Here's how the part is built. I have some questions about the finished solid (model axes, mm). Round coordinates to 2 decimals unless told otherwise and drop trailing zeros. Order: outer loops, then holes, each group sorted by start corner. A loop starts at its lowest first (then second) coordinate and runs counter-clockwise, first axis right, second up.
```python
from build123d import *

# Parameters (mm, degrees)
SKETCH_R        = 17.65
SKETCH_R_2      = 15.4
PAD_DEPTH       = 30
CHAMFER_SIZE    = 1.4
CHAMFER001_SIZE = 1.4


with BuildPart() as part:
    # Sketch → Pad (new body)
    with BuildSketch(Plane.XY):
        Circle(SKETCH_R)
        Circle(SKETCH_R_2, mode=Mode.SUBTRACT)
    extrude(amount=PAD_DEPTH)

    # Chamfer
    chamfer_edges = [part.edges().sort_by_distance(p)[0] for p in [
        (-17.65, 0, 30),
    ]]
    chamfer(chamfer_edges, length=CHAMFER_SIZE)

    # Chamfer001
    chamfer001_edges = [part.edges().sort_by_distance(p)[0] for p in [
        (-15.4, 0, 0),
    ]]
    chamfer(chamfer001_edges, length=CHAMFER001_SIZE)


solid = part.part
```
1) I need wall thicknesses on line 1 (Y direction, x = 0, z = 10); line 2 (Y direction, x = -6.5, z = 18.5); line 3 (X direction, y = 7.5, z = 8.75). Which ranges of each line are inside material? Lowest first, please.
2) If we section it at C-C (z = 20.5): Write out the boundary of the cut face in (x, y).
3) If we section it at A-A (y = 0): Write out the boundary of the cut face in (x, z), plus the area to 3 significant figures.
4) I'm going to push flat-ended pins straight in: pin 1 (1 mm diameter, centred on x = 11.5, z = 21, fed in from -Y); pin 2 (4 mm diameter, centred on y = -13.5, z = 11.5, fed in from +X); pin 3 (1 mm diameter, centred on y = -1, z = 7.5, fed in from +X). Where does each tip first touch, or does it pass through?
5) We'd pull the mould along X, two halves only. Please class faces 1 (the cylindrical face through (-14.006, -10.74, 14.1)), 2 (the cylindrical face through (-3.338, -15.034, 15.5)), 3 (the flat face through (6, -16, 0)): +X half, -X half, draft (parallel to the pull), parting line (faces both ways), or undercut.
Solutions:
1. line 1: y = -17.65 to -15.4, 15.4 to 17.65
1. line 2: y = -16.41 to -13.96, 13.96 to 16.41
1. line 3: x = -15.98 to -13.45, 13.45 to 15.98
2. outline: circle Ø35.3 at (0, 0); hole circle Ø30.8 at (0, 0)
3. outline: (-17.65, 0) - (-16.8, 0) - (-15.4, 1.4) - (-15.4, 30) - (-16.25, 30) - (-17.65, 28.6) - close; (15.4, 1.4) - (16.8, 0) - (17.65, 0) - (17.65, 28.6) - (16.25, 30) - (15.4, 30) - close
3. area: 131 mm2
4. pin 1: stops at y = -13.8
4. pin 2: stops at x = 13.39
4. pin 3: stops at x = 17.64
5. face 1: parting line
5. face 2: undercut
5. face 3: draft
